Verification items for the finished model (mm, model axes). A direction names the side the tool comes from. Coordinates: 2 decimals unless noted, no trailing zeros. Order: outer loops, then holes, each group sorted by start corner. A loop starts at its lowest first (then second) coordinate and runs counter-clockwise, first axis right, second up.
Q1. Thickness scan on line 1 (Z direction, x = -4.5, y = 4.5) (3 decimals); line 2 (Z direction, x = -5.75, y = -3.5); line 3 (Y direction, x = 1.25, z = 6). Record the ranges inside material, lowest first.
Q2. Set-up check for faces 1 (the flat face through (4, 0, 12.7)), 2 (the cylindrical face through (-0.69, 3.1, -1.57)), 3 (the cylindrical face through (6.513, -6.95, 6.261)): record each of +Z, -Z, +X, -X, +Y, -Y from which the full face is reachable in a straight line by a thin tool's end or side.
Q3. Depth check by flat-ended pin: P1, Ø4, axis at x = -3.5, z = 9, coming from the -Y side; P2, Ø2, axis at x = -7, y = 0.5, coming from the +Z side; P3, Ø5, axis at x = 2, y = 6.5, coming from the -Z side. Enter the tip coordinate at first touch or a pass-through.
Q4. Cross-section at B-B, the plane x = 7.75. Record the boundary of the cut face in (y, z), and give its area (3 significant figures).
Q5. Cross-section at D-D, the plane z = 2. Record the boundary of the cut face in (x, y) (3 decimals).
Q6. Cross-section at A-A, the plane z = 5. Record the boundary of the cut face in (x, y) (3 decimals), and give its area (3 significant figures).
Q7. Draft check along Y on faces 4 (the flat face through (-3.41, 5.75, 3.44)), 5 (the flat face through (4, 0, 0)), 6 (the cylindrical face through (-0.69, -3.1, 14.27)), 7 (the flat face through (4.4, -4.4, 6.4)). Enter one of: pulls with the +Y half, pulls with the -Y half, needs draft (parallel to the pull), parting line crosses it, or undercut.
Q8. Cross-section at C-C, the plane y = 8. Record the boundary of the cut face in (x, z).
from build123d import *

# Parameters (mm, degrees)
F0_R     = 9.525
F1_DEPTH = 12.7
F2_R     = 3.175
F3_DEPTH = 3.175
F4_R     = 3.175
F5_DEPTH = 3.175
F7_DEPTH = 25.4
F8_R     = 3.175
F9_DEPTH = 12.7


with BuildPart() as f1:
    # F0 (on Top) → F1 (new body)
    with BuildSketch(Plane.XY):
        Circle(F0_R)
    extrude(amount=F1_DEPTH)

    # F2 (on face) → F3 (join)
    with BuildSketch(Plane(origin=(0, 0, 0), x_dir=(1, 0, 0), z_dir=(0, 0, -1))):
        Circle(F2_R)
    extrude(amount=F3_DEPTH)

    # F4 (on face) → F5 (join)
    with BuildSketch(Plane.XY.offset(12.7)):
        Circle(F4_R)
    extrude(amount=F5_DEPTH)

    # F6 (on face) → F7 (cut)
    with BuildSketch(Plane(origin=(0, 0, 0), x_dir=(1, 0, 0), z_dir=(0, 0, -1))):
        with BuildLine():
            Line((0.360091, -9.518191), (0, -9.1581))
            Line((0, -9.1581), (0, -9.525))
            ThreePointArc((0, -9.525), (0.180078, -9.523298), (0.360091, -9.518191))
        make_face()
        with BuildLine():
            Line((0, -9.525), (0, -9.1581))
            Line((0, -9.1581), (-4.57905, -4.57905))
            Line((-4.57905, -4.57905), (-9.1581, 0))
            Line((-9.1581, 0), (-9.525, 0))
            ThreePointArc((-9.525, 0), (-6.735192, -6.735192), (0, -9.525))
        make_face()
        with BuildLine():
            Line((-9.525, 0), (-9.1581, 0))
            Line((-9.1581, 0), (-9.518191, 0.360091))
            ThreePointArc((-9.518191, 0.360091), (-9.523298, 0.180078), (-9.525, 0))
        make_face()
    extrude(amount=-F7_DEPTH, mode=Mode.SUBTRACT)

    # F8 (on face) → F9 (cut)
    with BuildSketch(Plane(origin=(-4.57905, 4.57905, 0), x_dir=(-0.707107, -0.707107, 0), z_dir=(-0.707107, 0.707107, 0))):
        with Locations((0, 6.35)):
            Circle(F8_R)
    extrude(amount=-F9_DEPTH, mode=Mode.SUBTRACT)


solid = f1.part
Check values:
1. line 1: z = 0 to 3.175, 9.525 to 12.7
1. line 2: z = 0 to 12.7
1. line 3: y = -9.44 to -5.71, 3.21 to 9.44
2. face 1: +Z
2. face 2: -Z
2. face 3: +Z, -Z
3. P1: stops at y = -9.41
3. P2: stops at z = 12.7
3. P3: stops at z = 0
4. outline: (-5.54, 0) - (5.54, 0) - (5.54, 12.7) - (-5.54, 12.7) - close
4. area: 141 mm2
5. outline: (-9.518, -0.36) arc R9.525 ccw (long way) to (0.36, 9.518) - close
6. outline: (-9.518, -0.36) arc R9.525 ccw (long way) to (0.36, 9.518) - (-2.547, 6.611) - (6.433, -2.369) - (2.369, -6.433) - (-6.611, 2.547) - close
6. area: 183 mm2
7. face 4: pulls with the +Y half
7. face 5: needs draft
7. face 6: parting line crosses it
7. face 7: undercut
8. outline: (-1.16, 0) - (5.17, 0) - (5.17, 12.7) - (-1.16, 12.7) - close
